```python
from build123d import *

# Parameters (mm, degrees)
F0_W     = 27.141710973
F0_H     = 25
F0_R     = 2
F2_DEPTH = 25
F1_W     = 8
F1_H     = 10
F4_R     = 1
F5_W     = 175
F5_H     = 25
F6_DEPTH = 25


# Not quite as in the source:
# - a feature names something its author has since deleted; it is built from what else it names


with BuildPart() as f2:
    # F0 (on Top) → F2 (new body)
    with BuildSketch(Plane.XY):
        with BuildLine():
            ThreePointArc((-61, 0), (-59.6453869522, 12.7838888967), (-55.641710973, 25))
            Line((-55.641710973, 25), (-61, 25))
            Line((-61, 25), (-61, 0))
        make_face()
        with BuildLine():
            Line((-59.5, 19.1311264697), (-59.5, 23.5))
            Line((-59.5, 23.5), (-57.9137289423, 23.5))
            ThreePointArc((-57.9137289423, 23.5), (-58.7474910104, 21.3303141089), (-59.5, 19.1311264697))
        make_face(mode=Mode.SUBTRACT)
        with BuildLine():
            ThreePointArc((-55.641710973, -25), (-59.6453869522, -12.7838888967), (-61, 0))
            Line((-61, 0), (-61, -25))
            Line((-61, -25), (-55.641710973, -25))
        make_face()
        with BuildLine():
            Line((-57.9137289423, -23.5), (-59.5, -23.5))
            Line((-59.5, -23.5), (-59.5, -19.1311264697))
            ThreePointArc((-59.5, -19.1311264697), (-58.7474910104, -21.3303141089), (-57.9137289423, -23.5))
        make_face(mode=Mode.SUBTRACT)
        with Locations((-74.5708554865, -12.5)):
            Rectangle(F0_W, F0_H)
        with Locations((-80.891710973, -12.5)):
            Circle(F0_R, mode=Mode.SUBTRACT)
        with Locations((-74.5708554865, 12.5)):
            Rectangle(F0_W, F0_H)
        with Locations((-80.891710973, 12.5)):
            Circle(F0_R, mode=Mode.SUBTRACT)
        with BuildLine():
            Line((-57.9137289423, 23.5), (-59.5, 23.5))
            Line((-59.5, 23.5), (-59.5, 19.1311264697))
            ThreePointArc((-59.5, 19.1311264697), (-58.7474910104, 21.3303141089), (-57.9137289423, 23.5))
        make_face()
        with BuildLine():
            Line((-59.5, -19.1311264697), (-59.5, -23.5))
            Line((-59.5, -23.5), (-57.9137289423, -23.5))
            ThreePointArc((-57.9137289423, -23.5), (-58.7474910104, -21.3303141089), (-59.5, -19.1311264697))
        make_face()
    extrude(amount=F2_DEPTH)

    # F1 (on Front) → F3 (revolve, cut)
    with BuildSketch(Plane.XZ):
        with Locations((-61, 12.5)):
            Rectangle(F1_W, F1_H)
    revolve(axis=Axis((0, 0, 15.2043728158), (0, 0, 1)), mode=Mode.SUBTRACT)

    # F4
    f4_edges = [f2.edges().sort_by_distance(p)[0] for p in [
        (-55.641711, 25, 21.25),
        (-55.641711, 25, 3.75),
        (-55.641711, -25, 3.75),
        (-55.641711, -25, 21.25),
    ]]
    fillet(f4_edges, radius=F4_R)

    # F5 (on Front) → F6 (intersect, symmetric)
    with BuildSketch(Plane.XZ):
        Rectangle(F5_W, F5_H)
    extrude(amount=F6_DEPTH, both=True, mode=Mode.INTERSECT)


solid = f2.part
```
Read the model definition and answer for the solid it produces. Units are mm, in the model's axes. A direction names the side the tool comes from. Coordinates: 2 decimals unless noted, no trailing zeros. Order: outer loops, then holes, each group sorted by start corner. A loop starts at its lowest first (then second) coordinate and runs counter-clockwise, first axis right, second up. Notation, with made-up numbers: (53, -25) - (64, -25) arc R31 cw to (64, 2) - close; hole circle Ø6 at (38.5, -15). An arc over 180 degrees is marked (long way). Answer as a JSON object with one key per item and string values. Group by question number.
Item 1: A tool of negligible diameter and unlimited length cuts with its end or side. For faces 1 (the face through (-62, 0, 7.5)), 2 (the face through (-78.984, 13.101, 6.162)), from which of +Z, -Z, +X, -X, +Y, -Y can it reach the whole face along a straight path? Write none if from no direction.
Item 2: The mould has two halves that part along Y. Classify faces 3 (the face through (-61, 0, 4)), 4 (the face through (-73, -25, 6)), 5 (the face through (-87.5, 0, 6)): +Y half, -Y half, draft (parallel to the pull), parting line (faces both ways), or undercut.
Item 3: Section C-C (y = -13.5) is taken. Give the vertices of the cut face in (x, z), plus the area to 3 significant figures.
Item 4: Consider probe 1 along Y at (x, z) = (-82, 4.75); probe 2 along Y at (x, z) = (-80, 8); probe 3 along Z at (x, y) = (-61.5, -6). Determine where each line is inside the solid, lowest interval first. Write a range as from..to.
Item 5: A flat-ended cylindrical pin translates along its axis: P1, Ø1, axis at x = -62.5, y = -12.5, coming from the +Z side. Find the tip coordinate at first contact, or state that the pin passes through.
Item 6: Section D-D (x = -63) is taken. Give the vertices of the cut face in (y, z), plus the area to 3 significant figures.
Item 7: Section B-B (x = -81.5) is taken. Give the vertices of the cut face in (y, z), plus the area to 3 significant figures.
Item 8: Section A-A (z = 9.5) is taken. Give the vertices of the cut face in (x, y).
Results are:
{
 "1": {"face 1": "+Z, +X", "face 2": "+Z, -Z"},
 "2": {"face 3": "undercut", "face 4": "-Y half", "face 5": "draft"},
 "3": {"outline": "(-87.5, 0) - (-82.62, 0) - (-82.62, 12.5) - (-87.5, 12.5) - close; (-79.16, 0) - (-59.49, 0) - (-59.49, 7.5) - (-63.58, 7.5) - (-63.58, 12.5) - (-79.16, 12.5) - close", "area": "286 mm^2"},
 "4": {"probe 1": "y = -25..-14.16, -10.84..10.84, 14.16..25", "probe 2": "y = -25..-14.29, -10.71..10.71, 14.29..25", "probe 3": "z = 0..7.5"},
 "5": {"P1": "stops at z = 7.5"},
 "6": {"outline": "(-25, 0) - (25, 0) - (25, 12.5) - (16, 12.5) - (16, 7.5) - (-16, 7.5) - (-16, 12.5) - (-25, 12.5) - close", "area": "465 mm^2"},
 "7": {"outline": "(-25, 0) - (-14.41, 0) - (-14.41, 12.5) - (-25, 12.5) - close; (-10.59, 0) - (10.59, 0) - (10.59, 12.5) - (-10.59, 12.5) - close; (14.41, 0) - (25, 0) - (25, 12.5) - (14.41, 12.5) - close", "area": "530 mm^2"},
 "8": {"outline": "(-87.5, -25) - (-60, -25) arc R65 cw to (-60, 25) - (-87.5, 25) - close; hole circle Ø4 at (-80.89, -12.5); hole circle Ø4 at (-80.89, 12.5)"}
}
